Can you work these out from the model? Positions are in its coordinate system, mm. Face numbers are marked on the shaded views. A direction names the side the tool comes from. Give positions to 0.01 mm unless a question says otherwise; leave off trailing zeros. Order: outer loops, then holes, each group sorted by start corner. A loop starts at its lowest first (then second) coordinate and runs counter-clockwise, first axis right, second up. Notation, with made-up numbers: (8, -5) - (46, -5) arc R35 ccw to (46, 33) - close; hole circle Ø5 at (7.5, -21). An arc over 180 degrees is marked (long way). One line per question, with ' | ' between items.
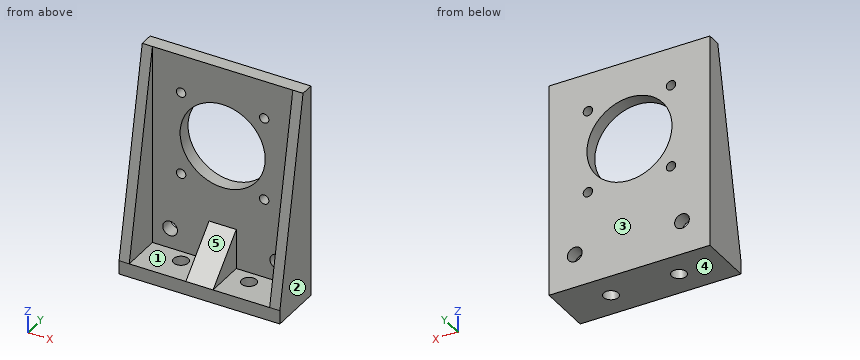
Autodesk Inventor part; units mm, degrees
ref_plane "YZ Plane" through (0, 0, 0) normal (1, 0, 0) x (0, 1, 0)
ref_plane "XZ Plane" through (0, 0, 0) normal (0, 1, 0) x (-1, 0, 0)
ref_plane "XY Plane" through (0, 0, 0) normal (0, 0, 1) x (1, 0, 0)
sketch "Sketch1" plane through (0, 0, 0) normal (0, 0, 1) x (1, 0, 0)
  line L0 (0, -1.25) -> (250, -1.25) construction
  line L1 (0, -1.25) -> (0, -6.4)
  line L2 (0, -6.4) -> (250, -6.4) construction
  line L3 (250, -1.25) -> (250, -6.4)
  line L4 (250, -18.75) -> (0, -18.75) construction
  line L5 (250, -13.6) -> (250, -18.75)
  line L6 (0, -13.6) -> (250, -13.6) construction
  line L7 (0, -13.6) -> (0, -18.75)
  line L8 (0, -20) -> (250, -20) construction
  line L9 (250, 0) -> (0, 0) construction
  line L10 (24.6484, -20) -> (84.6484, -20)
  line L11 (84.6484, -20) -> (84.6484, 0)
  line L12 (84.6484, 0) -> (24.6484, 0)
  line L13 (24.6484, 0) -> (24.6484, -20)
  line L14 (54.6484, -20) -> (54.6484, 0) construction
  circle A0 centre (67.3484, -10) radius 2.75
  circle A1 centre (41.9484, -10) radius 2.75
  line L15 (54.6484, -10) -> (41.9484, -10) construction
  line L16 (54.6484, -10) -> (67.3484, -10) construction
  point P0 (0, 0)
  dimension "d0" = 60
  dimension "d1" = 5.5
  dimension "d2" = 5.5
  dimension "d11" = 12.7
extrude "Extrusion1" add sketch "Sketch1" along normal blind 5.08
sketch "Sketch2" plane through (0, 0, 5.08) normal (0, 0, 1) x (1, 0, 0)
  line L0 (84.6484, 0) -> (24.6484, 0)
  line L1 (84.6484, -20) -> (84.6484, 0)
  line L2 (24.6484, 0) -> (84.6484, 0)
  line L3 (84.6484, 0) -> (84.6484, -5.08)
  line L4 (84.6484, -5.08) -> (24.6484, -5.08)
  line L5 (24.6484, -5.08) -> (24.6484, 0)
  point P0 (0, 0)
  dimension "d5" = 5.08
extrude "Extrusion2" add sketch "Sketch2" along normal blind 14.92
sketch "Sketch3" plane through (24.6484, -5.08, 5.08) normal (0, -1, 0) x (1, 0, 0)
  line L0 (0, -5.08) -> (0, 14.92)
  line L1 (0, 0) -> (60, 0)
  line L2 (0, 14.92) -> (0, 0)
  line L3 (60, -5.08) -> (60, 14.92)
  line L4 (19.1525, 952.0343) -> (19.1525, -47.9657) construction
  line L5 (19.1525, 952.0343) -> (14.0025, 952.0343)
  line L6 (14.0025, 952.0343) -> (14.0025, -47.9657) construction
  line L7 (19.1525, -47.9657) -> (14.0025, -47.9657)
  line L8 (1.6525, -47.9657) -> (1.6525, 952.0343) construction
  line L9 (6.8025, -47.9657) -> (1.6525, -47.9657)
  line L10 (6.8025, 952.0343) -> (6.8025, -47.9657) construction
  line L11 (6.8025, 952.0343) -> (1.6525, 952.0343)
  line L12 (0, 7.46) -> (1.6525, 7.46)
  line L13 (6.8025, 7.46) -> (14.0025, 7.46) construction
  line L14 (41.6525, -47.9657) -> (41.6525, 952.0343) construction
  line L15 (41.6525, -47.9657) -> (46.8025, -47.9657)
  line L16 (46.8025, -47.9657) -> (46.8025, 952.0343) construction
  line L17 (41.6525, 952.0343) -> (46.8025, 952.0343)
  line L18 (59.1525, 952.0343) -> (59.1525, -47.9657) construction
  line L19 (54.0025, 952.0343) -> (59.1525, 952.0343)
  line L20 (54.0025, -47.9657) -> (54.0025, 952.0343) construction
  line L21 (54.0025, -47.9657) -> (59.1525, -47.9657)
  line L22 (46.8025, 7.46) -> (54.0025, 7.46) construction
  line L23 (59.1525, 7.46) -> (60, 7.46)
  circle A0 centre (50.4025, 7.46) radius 2.75
  circle A1 centre (10.4025, 7.46) radius 2.75
  point P0 (-24.6484, -5.08)
  dimension "d8" = 5.5
extrude "Extrusion3" cut sketch "Sketch3" against normal blind 14.92
sketch "Sketch4" plane through (84.6484, -20, 0) normal (1, 0, 0) x (0, 0, -1)
  line L0 (-5.08, 0) -> (-5.08, 14.92)
  line L1 (-5.08, 14.92) -> (-20, 14.92)
  line L2 (-5.08, 0) -> (-20, 14.92)
  line L3 (-20, 14.92) -> (-5.08, 14.92)
  line L4 (-5.08, 14.92) -> (-5.08, 0)
  point P0 (0, 20)
extrude "Extrusion4" add sketch "Sketch4" against normal up to surface (60 mm away)
sketch "Sketch5" plane through (0, 0, 20) normal (0, 0, 1) x (1, 0, 0)
  line L0 (32.3009, 0) -> (37.8009, 0)
  line L1 (72.3009, 0) -> (77.8009, 0)
  circle A0 centre (41.9484, -10) radius 2.75
  circle A1 centre (67.3484, -10) radius 2.75
  line L2 (84.6484, 0) -> (24.6484, 0)
  line L3 (54.6484, 0) -> (54.6484, -20)
  line L4 (24.6484, -20) -> (84.6484, -20)
  line L5 (59.7284, -20) -> (49.5684, -20)
  line L6 (49.5684, -20) -> (49.5684, 0)
  line L7 (49.5684, 0) -> (59.7284, 0)
  line L8 (59.7284, 0) -> (59.7284, -20)
  line L9 (59.7284, -20) -> (49.5684, 0) construction
  line L10 (49.5684, -20) -> (59.7284, 0) construction
  line L11 (84.6484, -20) -> (82.1084, -20)
  line L12 (82.1084, -20) -> (82.1084, 0)
  line L13 (82.1084, 0) -> (84.6484, 0)
  line L14 (84.6484, 0) -> (84.6484, -20)
  line L15 (24.6484, -20) -> (27.1884, -20)
  line L16 (27.1884, -20) -> (27.1884, 0)
  line L17 (27.1884, 0) -> (24.6484, 0)
  line L18 (24.6484, 0) -> (24.6484, -20)
  line L19 (24.6484, -5.08) -> (84.6484, -5.08)
  line L20 (84.6484, 0) -> (24.6484, 0)
  line L21 (24.6484, 0) -> (24.6484, -5.08)
  line L22 (24.6484, -5.08) -> (84.6484, -5.08)
  line L23 (84.6484, -5.08) -> (84.6484, 0)
  line L24 (59.7284, -20) -> (82.1084, -20)
  line L25 (82.1084, -20) -> (82.1084, -5.08)
  line L26 (82.1084, -5.08) -> (59.7284, -5.08)
  line L27 (59.7284, -5.08) -> (59.7284, -20)
  line L28 (27.1884, -20) -> (49.5684, -20)
  line L29 (49.5684, -20) -> (49.5684, -5.08)
  line L30 (49.5684, -5.08) -> (27.1884, -5.08)
  line L31 (27.1884, -5.08) -> (27.1884, -20)
  line L32 (49.5684, -5.08) -> (12.5322, -5.08)
  line L33 (12.5322, -5.08) -> (12.5322, -38.5786)
  line L34 (12.5322, -38.5786) -> (49.5684, -38.5786)
  line L35 (49.5684, -38.5786) -> (49.5684, -5.08)
  line L36 (59.7284, -5.08) -> (93.4749, -5.08)
  line L37 (93.4749, -5.08) -> (93.4749, -31.7372)
  line L38 (93.4749, -31.7372) -> (59.7284, -31.7372)
  line L39 (59.7284, -31.7372) -> (59.7284, -5.08)
  point P0 (0, 0)
  point P1 (54.6484, -10)
  dimension "d14" = 2.54
  dimension "d15" = 2.54
  dimension "d16" = 10.16
extrude "Extrusion5" cut sketch "Sketch5" against normal blind 14.92 contours L19 L6 L4 L16 | L16 L4 L18 L19 | L18 L4 L35 L34 L33 L32 | L19 L12 L4 L8 | L4 L14 L36 L37 L38 L39 | L19 L14 L4 L12 | A0 | A1
sketch "Sketch8" plane through (24.6484, 0, 0) normal (0, 1, 0) x (1, 0, 0)
  line L0 (60, 0) -> (0, 0)
  line L1 (30, 0) -> (30, -133.2692) construction
  line L2 (0, -20) -> (0, -5.08)
  line L3 (0, -20) -> (60, -20)
  line L4 (60, -20) -> (60, -80)
  line L5 (60, -80) -> (0, -80)
  line L6 (0, -80) -> (0, -20)
  circle A0 centre (30, -50.2728) radius 15.875
  line L7 (45.5, -65.7728) -> (14.5, -65.7728) construction
  line L8 (14.5, -65.7728) -> (14.5, -34.7728) construction
  line L9 (14.5, -34.7728) -> (45.5, -34.7728) construction
  line L10 (45.5, -34.7728) -> (45.5, -65.7728) construction
  line L11 (45.5, -65.7728) -> (14.5, -34.7728) construction
  line L12 (14.5, -65.7728) -> (45.5, -34.7728) construction
  circle A1 centre (14.5, -65.7728) radius 1.75
  circle A2 centre (14.5, -34.7728) radius 1.75
  circle A3 centre (45.5, -34.7728) radius 1.75
  circle A4 centre (45.5, -65.7728) radius 1.75
  point P0 (-24.6484, 0)
  dimension "d24" = 31
  dimension "d25" = 31.75
  dimension "d26" = 3.5
extrude "Extrusion8" add sketch "Sketch8" against normal up to surface (5.08 mm away)
sketch "Sketch10" plane through (24.6484, -5.08, 5.08) normal (0, -1, 0) x (1, 0, 0)
  line L0 (0, 0) -> (24.92, 0)
  line L1 (0, 0) -> (3.81, 0)
  line L2 (3.81, 0) -> (3.81, 74.92)
  line L3 (3.81, 74.92) -> (0, 74.92)
  line L4 (0, 74.92) -> (0, 0)
  line L5 (60, 74.92) -> (60, 0)
  line L6 (35.08, 0) -> (60, 0)
  line L7 (60, 74.92) -> (56.19, 74.92)
  line L8 (56.19, 74.92) -> (56.19, 0)
  line L9 (56.19, 0) -> (60, 0)
  line L10 (60, 0) -> (60, 74.92)
  point P0 (-24.6484, -5.08)
  dimension "d29" = 3.81
extrude "Extrusion9" add sketch "Sketch10" along normal up to surface (14.92 mm away)
sketch "Sketch11" plane through (84.6484, -20, 0) normal (1, 0, 0) x (0, 0, -1)
  line L0 (-80, 0) -> (-5.08, 0)
  line L1 (-5.08, 14.92) -> (-5.08, 0)
  line L2 (-80, 14.92) -> (-5.08, 14.92)
  line L3 (-80, 14.92) -> (-80, 0)
  line L4 (-5.08, 0) -> (-80, 14.92)
  point P0 (0, 20)
extrude "Extrusion10" cut sketch "Sketch11" against normal through all contours L3 L4 L0
properties part number "double90andMotor"
(1) Imagine slicing it at A-A (x = 62). List the corners of the cut face in (y, z) for me.
Answer below:
outline: (-20, 0) - (0, 0) - (0, 36.2) - (-5.08, 36.2) - (-5.08, 5.08) - (-20, 5.08) - close; (-5.08, 64.34) - (0, 64.34) - (0, 80) - (-5.08, 80) - close
(2) If we mould it in two halves opening along X, with no side actions, what happens to the marked faces 1, 2 and 3? For each: released by +X, released by -X, zero draft, split by the parting line, or undercut.
Answer below:
face 1: undercut | face 2: released by +X | face 3: zero draft
(3) On a 3-axis mill with a long thin cutter (end or side, diameter ignored), from which of +Z, -Z, +X, -X, +Y, -Y can I reach the whole of each face in a straight line? I mean the marked faces 4 and 5. Say none if no direction works.
Answer below:
face 4: -Z, +X, -X, +Y, -Y | face 5: +Z, -Y
(4) Imagine slicing it at B-B (z = 12.54). List the corners of the cut face in (x, y) for me.
Answer below:
outline: (24.65, -18.51) - (28.46, -18.51) - (28.46, -5.08) - (32.3, -5.08) - (32.3, 0) - (24.65, 0) - close; (37.8, -5.08) - (49.57, -5.08) - (49.57, -12.54) - (59.73, -12.54) - (59.73, -5.08) - (72.3, -5.08) - (72.3, 0) - (37.8, 0) - close; (77.8, -5.08) - (80.84, -5.08) - (80.84, -18.51) - (84.65, -18.51) - (84.65, 0) - (77.8, 0) - close
(5) If I drill on line 1 (X direction, y = -9.5, z = 11); line 2 (X direction, y = -12.25, z = 33.5); line 3 (Z direction, x = 71, y = -4), over which ranges is the centre line in solid material (lowest first)?
Answer below:
line 1: 24.65 to 28.46, 49.57 to 59.73, 80.84 to 84.65 | line 2: 24.65 to 28.46, 80.84 to 84.65 | line 3: 0 to 33.24, 36.3 to 64.24, 67.3 to 80
(6) Imagine slicing it at C-C (y = -10). List the corners of the cut face in (x, z) for me, and give its area (3 significant figures).
Answer below:
outline: (24.65, 0) - (39.2, 0) - (39.2, 5.08) - (28.46, 5.08) - (28.46, 55.29) - (24.65, 55.29) - close; (44.7, 0) - (64.6, 0) - (64.6, 5.08) - (59.73, 5.08) - (59.73, 15.08) - (49.57, 15.08) - (49.57, 5.08) - (44.7, 5.08) - close; (70.1, 0) - (84.65, 0) - (84.65, 55.29) - (80.84, 55.29) - (80.84, 5.08) - (70.1, 5.08) - close | area: 733 mm^2
(7) Imagine slicing it at D-D (z = 55.5). List the corners of the cut face in (x, y) for me.
Answer below:
outline: (24.65, -9.96) - (28.46, -9.96) - (28.46, -5.08) - (39.66, -5.08) - (39.66, 0) - (24.65, 0) - close; (69.64, -5.08) - (80.84, -5.08) - (80.84, -9.96) - (84.65, -9.96) - (84.65, 0) - (69.64, 0) - close
(8) Will these pins go through, and if not, where does the flat tip stop? pin 1 (2 mm diameter, centred on x = 70.15, z = 65.77, fed in from -Y); pin 2 (6.5 mm diameter, centred on x = 75.05, z = 12.54, fed in from -Y); pin 3 (12 mm diameter, centred on x = 41, y = -11.5, fed in from +Z); pin 4 (2 mm diameter, centred on x = 61, z = 14, fed in from +Y).
Answer below:
pin 1: through | pin 2: y = -5.08 | pin 3: z = 5.08 | pin 4: y = 0
